Part model, mm, in its own coordinate system. A direction names the side the tool comes from. Round coordinates to 2 decimals unless told otherwise and drop trailing zeros. Loops run counter-clockwise (first coordinate to the right, second up) from the corner with the lowest first, then second, coordinate; pieces in that order, holes last. Notation, with made-up numbers: (86, 14) - (119, 14) arc R27 cw to (119, 47) - close; hole circle Ø7 at (-11.75, 18). An arc over 180 degrees is marked (long way). Put each result on its own line as item: value.
from build123d import *

# Parameters (mm, degrees)
SCALE1_SCALE = 3.2


with BuildPart() as part:
    # Sketch1 → Revolve1 (revolve)
    with BuildSketch(Plane.XY):
        with BuildLine():
            Line((-4.5, 15.7), (-4.5, 7.8))
            ThreePointArc((-4.5, 7.8), (-4.412132034, 7.587867966), (-4.2, 7.5))
            Line((-4.2, 7.5), (4.2, 7.5))
            ThreePointArc((4.2, 7.5), (4.412132034, 7.587867966), (4.5, 7.8))
            Line((4.5, 7.8), (4.5, 15.7))
            ThreePointArc((4.5, 15.7), (4.412132034, 15.912132034), (4.2, 16))
            Line((4.2, 16), (-4.2, 16))
            ThreePointArc((-4.2, 16), (-4.412132034, 15.912132034), (-4.5, 15.7))
        make_face()
    revolve(axis=Axis((50, 0, 0), (-1, 0, 0)))

    # Sketch2 → Cut-Revolve1 (revolve, cut)
    with BuildSketch(Plane.XY):
        Polygon((-6.3, 7.5), (-4.5, 7.5), (-4.5, 10.22), (-4.48, 10.22), (-4.48, 12.08), (-4.3, 12.08), (-4.3, 13.28), (-6.3, 13.28), align=None)
    revolve(axis=Axis((50, 0, 0), (-1, 0, 0)), mode=Mode.SUBTRACT)

    # Sketch3 → Cut-Revolve2 (revolve, cut)
    with BuildSketch(Plane.XY):
        Polygon((4.3, 13.28), (4.3, 12.08), (4.48, 12.08), (4.48, 10.22), (4.5, 10.22), (4.5, 7.5), (6.3, 7.5), (6.3, 13.28), align=None)
    revolve(axis=Axis((50, 0, 0), (-1, 0, 0)), mode=Mode.SUBTRACT)


with BuildPart() as part_1:
    # Scale1: scaled about (0, 0, 0)
    add(part.part.scale(SCALE1_SCALE))


solid = part_1.part
1. Probe line 1 along Z through (x, y) = (-14.05, 0); line 2 along Y through (x, z) = (14.1, 0); line 3 along X through (y, z) = (-18, -29). List the from-to ranges inside material, lowest first. Write a range as [from, to].
A:
line 1: z = [-50.98, -42.5], [-38.66, -24.22], [24.22, 38.66], [42.5, 50.98]
line 2: y = [-50.94, -42.5], [-38.66, -24.26], [24.26, 38.66], [42.5, 50.94]
line 3: x = [-14.34, 14.34]
2. Pin check, flat tips, straight feed: P1, Ø2, axis at y = -37.5, z = 16.5, coming from the -X side; P2, Ø2, axis at x = 11.5, z = 5.5, coming from the -Y side; P3, Ø5, axis at x = -7.5, z = -23, coming from the -Y side; P4, Ø10, axis at y = -9, z = -12.5, coming from the +X side. Stop position of each tip, or through.
A:
P1: stops at x = -13.76
P2: stops at y = -51
P3: stops at y = -46.92
P4: passes through
3. Tool access for faces 1 (the cylindrical face through (-14.044, -8.38, 37.737)), 2 (the flat face through (13.76, 9, 38)): list every direction of +Z, -Z, +X, -X, +Y, -Y with a clear straight run to the whole face (end or side of a thin tool).
A:
face 1: -X
face 2: +X
4. Band-saw the part on A-A (x = -9.75). List the corners of the cut face in (y, z).
A:
outline: circle Ø102.4 at (0, 0); hole circle Ø48 at (0, 0)
5. Two-plate mould, pull along Y, no slides. Class faces 3 (the cylindrical face through (-0.188, -40.631, 31.154)), 4 (the cylindrical face through (14.08, 19.61, 37.7)): pulls with the +Y half, pulls with the -Y half, needs draft (parallel to the pull), parting line crosses it, or undercut.
A:
face 3: parting line crosses it
face 4: undercut
